Can you work these out from the drawing? Everything is in mm from the part's minimum corner. Coordinates: 2 decimals unless noted, no trailing zeros. Loops run counter-clockwise (first coordinate to the right, second up) from the corner with the lowest first, then second, coordinate; pieces in that order, holes last.
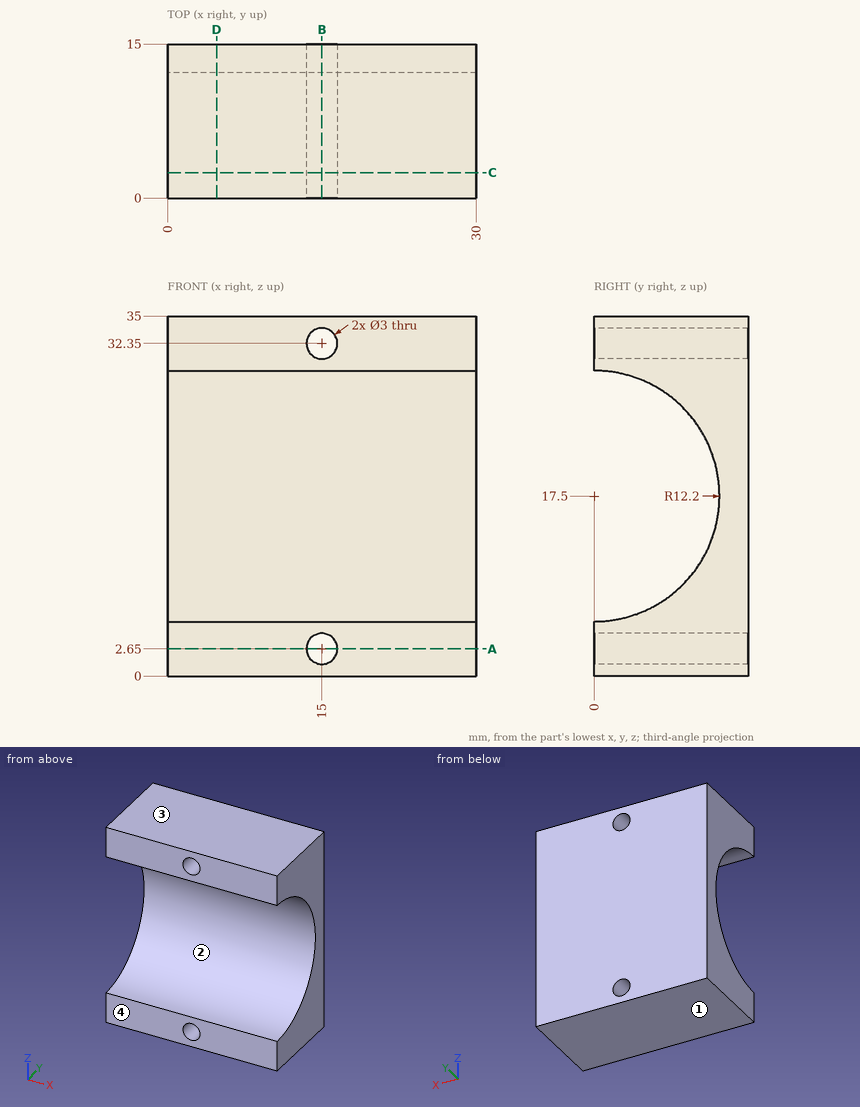
(1) Imagine slicing it at C-C, the plane y = 2.5. Write out the boundary of the cut face in (x, z).
Answers:
outline: (0, 0) - (30, 0) - (30, 5.56) - (0, 5.56) - close; (0, 29.44) - (30, 29.44) - (30, 35) - (0, 35) - close; hole circle Ø3 at (15, 2.65); hole circle Ø3 at (15, 32.35)
(2) Imagine slicing it at D-D, the plane x = 4.75. Write out the boundary of the cut face in (y, z), and give its area (3 significant figures).
Answers:
outline: (0, 0) - (15, 0) - (15, 35) - (0, 35) - (0, 29.7) arc R12.2 cw to (0, 5.3) - close
area: 291 mm2
(3) Imagine slicing it at B-B, the plane x = 15. Write out the boundary of the cut face in (y, z), and give its area (3 significant figures).
Answers:
outline: (0, 0) - (15, 0) - (15, 1.15) - (0, 1.15) - close; (0, 4.15) - (15, 4.15) - (15, 30.85) - (0, 30.85) - (0, 29.7) arc R12.2 cw to (0, 5.3) - close; (0, 33.85) - (15, 33.85) - (15, 35) - (0, 35) - close
area: 201 mm2
(4) Imagine slicing it at A-A, the plane z = 2.65. Write out the boundary of the cut face in (x, y), and give its area (3 significant figures).
Answers:
outline: (0, 0) - (13.5, 0) - (13.5, 15) - (0, 15) - close; (16.5, 0) - (30, 0) - (30, 15) - (16.5, 15) - close
area: 405 mm2
(5) For pin 1 (4 mm diameter, centred on x = 5.5, z = 9.5, fed in from -Y); pin 2 (2.5 mm diameter, centred on x = 15, z = 2.65, fed in from +Y), each with a flat end and sliding along its axis, tell me the tip position at first contact or that it passes through.
Answers:
pin 1: stops at y = 6.99
pin 2: passes through
(6) I need wall thicknesses on probe 1 along X at (y, z) = (7, 2.65); probe 2 along Z at (x, y) = (28.75, 4.5); probe 3 along Z at (x, y) = (20, 9). Which ranges of each line are inside material? Lowest first, please.
Answers:
probe 1: x = 0 to 13.5, 16.5 to 30
probe 2: z = 0 to 6.16, 28.84 to 35
probe 3: z = 0 to 9.26, 25.74 to 35
(7) We'd pull the mould along Z, two halves only. Please class the marked faces 1, 2, 3 and 4: +Z half, -Z half, draft (parallel to the pull), parting line (faces both ways), or undercut.
Answers:
face 1: -Z half
face 2: undercut
face 3: +Z half
face 4: draft
